Here's how the part is built. I have some questions about the finished solid (model axes, mm). A direction names the side the tool comes from. Coordinates: 2 decimals unless noted, no trailing zeros. Write each loop counter-clockwise with the first axis right and the second up, starting at its lowest first coordinate (ties: lowest second). Pieces come first, ordered by that corner, then holes. Notation, with made-up numbers: (11, 49.25) -> (62, 49.25) arc R27 cw to (62, 74.25) -> close; hole circle Ø9 at (43, 65). An arc over 180 degrees is marked (long way). Use a Markdown table: item, result. Add a question column.
Item 1: On a 3-axis mill with a long thin cutter (end or side, diameter ignored), from which of +Z, -Z, +X, -X, +Y, -Y can I reach the whole of each face in a straight line? I mean faces 1 (the flat face through (-70.816, -44.581, 6.334)), 2 (the flat face through (74.02, -39.04, 6.33)), 3 (the flat face through (3.2, 84, 6)). Say none if no direction works.
Item 2: If we mould it in two halves opening along Y, with no side actions, what happens to faces 4 (the cylindrical face through (-59.385, -39.494, 7.888)), 5 (the cylindrical face through (-63.9, -31.7, 7.9)), 6 (the flat face through (-3.2, 84, 6))? For each: pulls with the +Y half, pulls with the -Y half, needs draft (parallel to the pull), parting line crosses it, or undercut.
Item 3: If I drill on line 1 along X through (y, z) = (0, -12.5); line 2 along Y through (x, z) = (0, -4); line 3 along X through (y, z) = (13, -5), over which ranges is the centre line in solid material (lowest first)? Write a range as from..to.
Item 4: Imagine slicing it at B-B, the plane y = 77.5. Write out the boundary of the cut face in (x, z), and give its area (3 significant figures).
Item 5: Will these pins go through, and if not, where does the flat tip stop? pin 1 Ø1 at (x, y) = (48, 38) entering from -Z; pin 2 Ø10 at (x, y) = (36, 46) entering from -Z; pin 3 Ø13 at (y, z) = (87.5, 5) entering from -X; pin 4 Ø6 at (x, z) = (-25, 4.5) entering from +Y.
Item 6: Imagine slicing it at A-A, the plane z = 3. Write out the boundary of the cut face in (x, y), and give its area (3 significant figures).
Item 7: Imagine slicing it at C-C, the plane z = -10.5. Write out the boundary of the cut face in (x, y), and give its area (3 significant figures).
```python
from build123d import *

# Parameters (mm, degrees)
SKETCH_R              = 93
SKETCH_R_2            = 63
PAD_DEPTH             = 16
POCKET_DEPTH          = 543.060769
POLARPATTERN_COUNT    = 3
SKETCH002_W           = 32
SKETCH002_H           = 146
POCKET001_DEPTH       = 16.001
SKETCH003_R           = 2.6
POCKET002_DEPTH       = 546.51444
POLARPATTERN001_COUNT = 3
PAD001_DEPTH          = 16
FILLET_R              = 1
FILLET001_R           = 2
FILLET002_R           = 10
FILLET003_R           = 5


with BuildPart() as part:
    # Sketch → Pad (new body)
    with BuildSketch(Plane.XY):
        Circle(SKETCH_R)
        Circle(SKETCH_R_2, mode=Mode.SUBTRACT)
    extrude(amount=PAD_DEPTH)

    # Sketch001 (on Face4 of Pad) → Pocket (cut, through all)
    with BuildSketch(Plane.XY.offset(16)):
        with BuildLine():
            ThreePointArc((62.158402, -32.192128), (60.621778, 35), (3.2, 69.926819))
            Line((3.2, 205.926819), (3.2, 69.926819))
            ThreePointArc((179.937856, -100.192128), (178.359387, 102.97584), (3.2, 205.926819))
            Line((62.158402, -32.192128), (179.937856, -100.192128))
        make_face()
    pocket = extrude(amount=-POCKET_DEPTH, mode=Mode.SUBTRACT)

    # PolarPattern: Pocket ×3 about axis
    polarpattern_axis = Axis((0, 0, 16), (0, 0, 1))
    for i in range(1, POLARPATTERN_COUNT):
        add(pocket.rotate(polarpattern_axis, i * 360 / POLARPATTERN_COUNT), mode=Mode.SUBTRACT)

    # Sketch002 (on Face4 of PolarPattern) → Pocket001 (cut, through all)
    with BuildSketch(Plane.XY.offset(16)):
        with Locations((0, -73)):
            Rectangle(SKETCH002_W, SKETCH002_H)
    extrude(amount=-POCKET001_DEPTH, mode=Mode.SUBTRACT)

    # Sketch003 (on Face5 of Pocket001) → Pocket002 (cut, through all)
    with BuildSketch(Plane.YZ.offset(3.2)):
        with Locations((82.94493, 10)):
            Circle(SKETCH003_R)
    pocket002 = extrude(amount=-POCKET002_DEPTH, mode=Mode.SUBTRACT)

    # PolarPattern001: Pocket002 ×3 about axis
    polarpattern001_axis = Axis((0, 0, 0), (0, 0, 1))
    for i in range(1, POLARPATTERN001_COUNT):
        add(pocket002.rotate(polarpattern001_axis, i * 360 / POLARPATTERN001_COUNT), mode=Mode.SUBTRACT)

    # Sketch004 (on Face2 of PolarPattern001) → Pad001 (join)
    with BuildSketch(Plane(origin=(0, 0, 0), x_dir=(1, 0, 0), z_dir=(0, 0, -1))):
        with BuildLine():
            ThreePointArc((-16, 60.934391), (0, -63), (16, 60.934391))
            Line((16, 66.1469), (16, 60.934391))
            ThreePointArc((-16, 66.1469), (0, -68.054481), (16, 66.1469))
            Line((-16, 66.1469), (-16, 60.934391))
        make_face()
    extrude(amount=PAD001_DEPTH)

    # Fillet
    fillet_edges = [part.edges().sort_by_distance(p)[0] for p in [
        (0, 68.054481, 0),
    ]]
    fillet(fillet_edges, radius=FILLET_R)

    # Fillet001
    fillet001_edges = [part.edges().sort_by_distance(p)[0] for p in [
        (-16, -60.934391, -8),
        (-16, -60.934391, 8),
        (16, -60.934391, -8),
        (16, -60.934391, 8),
    ]]
    fillet(fillet001_edges, radius=FILLET001_R)

    # Fillet002
    fillet002_edges = [part.edges().sort_by_distance(p)[0] for p in [
        (-80.540363, -46.5, 0),
        (80.540363, -46.5, 0),
        (0, 93, 0),
    ]]
    fillet(fillet002_edges, radius=FILLET002_R)

    # Fillet003
    fillet003_edges = [part.edges().sort_by_distance(p)[0] for p in [
        (62.158402, -32.192128, 8),
        (58.958402, -37.734691, 8),
        (-58.958402, -37.734691, 8),
        (-62.158402, -32.192128, 8),
        (-3.2, 69.926819, 8),
        (3.2, 69.926819, 8),
    ]]
    fillet(fillet003_edges, radius=FILLET003_R)


solid = part.part
```
Ans:
| question | item | result |
|---|---|---|
| 1 | face 1 | +Z, -Z, -Y |
| 1 | face 2 | +Z, -Z, +X |
| 1 | face 3 | +Z, -Z, +X, +Y |
| 2 | face 4 | pulls with the -Y half |
| 2 | face 5 | undercut |
| 2 | face 6 | needs draft |
| 3 | line 1 | x = -68.05..-63, 63..68.05 |
| 3 | line 2 | y = 63..68.05 |
| 3 | line 3 | x = -66.8..-61.64, 61.64..66.8 |
| 4 | outline | (-3.2, 0) -> (3.2, 0) -> (3.2, 16) -> (-3.2, 16) -> close |
| 4 | area | 102 mm^2 |
| 5 | pin 1 | passes through |
| 5 | pin 2 | stops at z = -16 |
| 5 | pin 3 | stops at x = -3.2 |
| 5 | pin 4 | stops at y = 66.45 |
| 6 | outline | (-79.62, -42.27) arc R90.14 ccw to (-76.42, -47.81) -> (-62.96, -40.05) arc R5 cw to (-56.43, -41.42) arc R70 ccw to (-16, -68.15) -> (-16, -62.46) arc R2 ccw to (-17.45, -60.54) arc R63 cw (long way) to (17.45, -60.54) arc R2 ccw to (16, -62.46) -> (16, -68.15) arc R70 ccw to (56.43, -41.42) arc R5 cw to (62.96, -40.05) -> (76.42, -47.81) arc R90.14 ccw to (79.62, -42.27) -> (66.16, -34.5) arc R5 cw to (64.09, -28.16) arc R70 ccw to (7.65, 69.58) arc R5 cw to (3.2, 74.55) -> (3.2, 90.08) arc R90.14 ccw to (-3.2, 90.08) -> (-3.2, 74.55) arc R5 cw to (-7.65, 69.58) arc R70 ccw to (-64.09, -28.16) arc R5 cw to (-66.16, -34.5) -> close |
| 6 | area | 3,110 mm^2 |
| 7 | outline | (-17.45, -60.54) arc R63 cw (long way) to (17.45, -60.54) arc R2 ccw to (16, -62.46) -> (16, -66.15) arc R68.05 ccw (long way) to (-16, -66.15) -> (-16, -62.46) arc R2 ccw to start |
| 7 | area | 1,920 mm^2 |
